Input: part model. Units: mm. Frame: model coordinates. Coordinates: 2 decimals unless noted, no trailing zeros. Order: outer loops, then holes, each group sorted by start corner. A loop starts at its lowest first (then second) coordinate and runs counter-clockwise, first axis right, second up. Notation, with made-up numbers: (52.25, 19.5) - (70.25, 19.5) arc R23 cw to (70.25, 27.5) - close; hole circle Ø2 at (15.5, 44.5). An arc over 180 degrees is marked (long way). One line per question, with ' | ' between items. Start each with the question number.
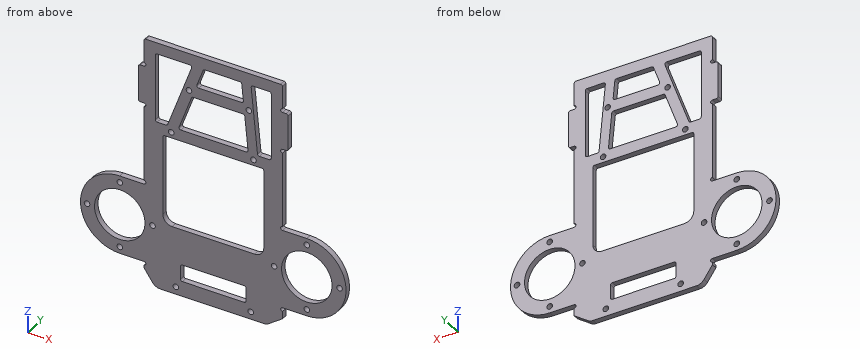
```python
from build123d import *
from OCP.BRepFilletAPI import BRepFilletAPI_MakeChamfer

# Parameters (mm, degrees)
SKETCH_1_R          = 13.5
SKETCH_1_R_2        = 1.5
EXTRUDE_1_DEPTH     = 3
SKETCH_3_W          = 54
SKETCH_3_H          = 48
SKETCH_3_W_2        = 35
SKETCH_3_H_2        = 9
CUT_EXTRUDE_2_DEPTH = 123.678441464
SKETCH_2_R          = 1
CUT_EXTRUDE_1_DEPTH = 123.678441464
CHAMFER_1_SIZE      = 6
CHAMFER_1_SIZE2     = 8.56888804
FILLET_1_R          = 1
FILLET_2_R          = 5


with BuildPart() as part:
    # 草图1 → 凸台-拉伸1 (new body)
    with BuildSketch(Plane(origin=(0, 0, 0), x_dir=(1, 0, 0), z_dir=(0, 1, 0))):
        with BuildLine():
            Line((-37, 21), (-50, 21))
            ThreePointArc((-50, 21), (-71, 0), (-50, -21))
            Line((-50, -21), (-37, -21))
            Line((-37, -21), (-37, -65))
            Line((-37, -65), (-40, -65))
            Line((-40, -65), (-40, -85))
            Line((-40, -85), (-37, -85))
            Line((-37, -85), (-37, -100))
            Line((-37, -100), (37, -100))
            Line((37, -100), (37, -85))
            Line((37, -85), (40, -85))
            Line((40, -85), (40, -65))
            Line((40, -65), (37, -65))
            Line((37, -65), (37, -21))
            Line((37, -21), (50, -21))
            ThreePointArc((50, -21), (71, 0), (50, 21))
            Line((50, 21), (37, 21))
            Line((37, 21), (37, 33))
            Line((37, 33), (-37, 33))
            Line((-37, 33), (-37, 21))
        make_face()
        with Locations(Location((-50, 0, 0), (0, 0, 270))):
            Circle(SKETCH_1_R, mode=Mode.SUBTRACT)
        with Locations(Location((50, 0, 0), (0, 0, 90))):
            Circle(SKETCH_1_R, mode=Mode.SUBTRACT)
        with Locations(Location((-50, 17.5, 0), (0, 0, 270))):
            Circle(SKETCH_1_R_2, mode=Mode.SUBTRACT)
        with Locations(Location((-32.5, 0, 0), (0, 0, 270))):
            Circle(SKETCH_1_R_2, mode=Mode.SUBTRACT)
        with Locations(Location((-67.5, 0, 0), (0, 0, 270))):
            Circle(SKETCH_1_R_2, mode=Mode.SUBTRACT)
        with Locations(Location((-50, -17.5, 0), (0, 0, 270))):
            Circle(SKETCH_1_R_2, mode=Mode.SUBTRACT)
        with Locations(Location((32.5, 0, 0), (0, 0, 270))):
            Circle(SKETCH_1_R_2, mode=Mode.SUBTRACT)
        with Locations(Location((50, -17.5, 0), (0, 0, 270))):
            Circle(SKETCH_1_R_2, mode=Mode.SUBTRACT)
        with Locations(Location((50, 17.5, 0), (0, 0, 270))):
            Circle(SKETCH_1_R_2, mode=Mode.SUBTRACT)
        with Locations(Location((67.5, 0, 0), (0, 0, 270))):
            Circle(SKETCH_1_R_2, mode=Mode.SUBTRACT)
        with Locations(Location((-20, 29, 0), (0, 0, 270))):
            Circle(SKETCH_1_R_2, mode=Mode.SUBTRACT)
        with Locations(Location((20, 29, 0), (0, 0, 90))):
            Circle(SKETCH_1_R_2, mode=Mode.SUBTRACT)
        with Locations(Location((21.5, -54, 0), (0, 0, 270))):
            Circle(SKETCH_1_R_2, mode=Mode.SUBTRACT)
        with Locations(Location((-13, -80, 0), (0, 0, 270))):
            Circle(SKETCH_1_R_2, mode=Mode.SUBTRACT)
        with Locations(Location((19, -80, 0), (0, 0, 270))):
            Circle(SKETCH_1_R_2, mode=Mode.SUBTRACT)
        with Locations(Location((-22.5, -54, 0), (0, 0, 270))):
            Circle(SKETCH_1_R_2, mode=Mode.SUBTRACT)
    extrude(amount=EXTRUDE_1_DEPTH)

    # 草图3 → 切除-拉伸2 (cut, through all)
    with BuildSketch(Plane(origin=(0, 3, 0), x_dir=(1, 0, 0), z_dir=(0, 1, 0))):
        with Locations((0, -27)):
            Rectangle(SKETCH_3_W, SKETCH_3_H)
        with Locations((0, 20.5)):
            Rectangle(SKETCH_3_W_2, SKETCH_3_H_2)
        Polygon((-24.597833201, -57), (-11.078602431, -94), (-31, -94), (-31, -57), align=None)
        Polygon((-18.742190282, -57), (18.700008099, -57), (16.776931176, -77), (-11.434497974, -77), align=None)
        Polygon((-9.242190282, -83), (-5.222959512, -94), (15.142315791, -94), (16.200008099, -83), align=None)
        Polygon((23.723068824, -57), (20.165376517, -94), (31, -94), (31, -57), align=None)
    extrude(amount=-CUT_EXTRUDE_2_DEPTH, mode=Mode.SUBTRACT)

    # 草图2 → 切除-拉伸1 (cut, through all)
    with BuildSketch(Plane(origin=(0, 3, 0), x_dir=(1, 0, 0), z_dir=(0, 1, 0))):
        with Locations((-37, 22)):
            Circle(SKETCH_2_R)
        with Locations((-37, -22)):
            Circle(SKETCH_2_R)
        with Locations((-37, -64)):
            Circle(SKETCH_2_R)
        with Locations((-37, -86)):
            Circle(SKETCH_2_R)
        with Locations((37, -86)):
            Circle(SKETCH_2_R)
        with Locations((37, -64)):
            Circle(SKETCH_2_R)
        with Locations((37, -22)):
            Circle(SKETCH_2_R)
        with Locations((37, 22)):
            Circle(SKETCH_2_R)
    extrude(amount=-CUT_EXTRUDE_1_DEPTH, mode=Mode.SUBTRACT)

    # 倒角1: one chamfer whose edges measure the first distance from different faces: ONE call of the kernel's chamfer builder (chamfer() names one face for all edges)
    chamfer_1_edges_1 = [part.edges().sort_by_distance(p)[0] for p in [
        (-37, 1.5, -33),
    ]]
    chamfer_1_side_1 = [part.faces().sort_by_distance(p)[0] for p in [
        (0, 1.5, -33),
    ]]
    chamfer_1_edges_2 = [part.edges().sort_by_distance(p)[0] for p in [
        (37, 1.5, -33),
    ]]
    chamfer_1_side_2 = [part.faces().sort_by_distance(p)[0] for p in [
        (37, 1.5, -28),
    ]]
    chamfer_1 = BRepFilletAPI_MakeChamfer(part.part.solid().wrapped)
    for e in chamfer_1_edges_1:
        chamfer_1.Add(CHAMFER_1_SIZE, CHAMFER_1_SIZE2, e.wrapped, chamfer_1_side_1[0].wrapped)  # the first distance lies on this face
    for e in chamfer_1_edges_2:
        chamfer_1.Add(CHAMFER_1_SIZE, CHAMFER_1_SIZE2, e.wrapped, chamfer_1_side_2[0].wrapped)  # the first distance lies on this face
    add(Compound.cast(chamfer_1.Shape()), mode=Mode.REPLACE)

    # 圆角1
    fillet_1_edges = [part.edges().sort_by_distance(p)[0] for p in [
        (23.723068824, 1.5, 57),
        (31, 1.5, 57),
        (31, 1.5, 94),
        (20.165376517, 1.5, 94),
        (-17.5, 1.5, -16),
        (-17.5, 1.5, -25),
        (17.5, 1.5, -25),
        (17.5, 1.5, -16),
        (-11.434497974, 1.5, 77),
        (-18.742190282, 1.5, 57),
        (18.700008099, 1.5, 57),
        (16.776931176, 1.5, 77),
        (-11.078602431, 1.5, 94),
        (-31, 1.5, 94),
        (-31, 1.5, 57),
        (-24.597833201, 1.5, 57),
        (-9.242190282, 1.5, 83),
        (16.200008099, 1.5, 83),
        (15.142315791, 1.5, 94),
        (-5.222959512, 1.5, 94),
        (-27, 1.5, 51),
        (27, 1.5, 51),
        (40, 1.5, 65),
        (40, 1.5, 85),
        (37, 1.5, 100),
        (-37, 1.5, 100),
        (-40, 1.5, 85),
        (-40, 1.5, 65),
    ]]
    fillet(fillet_1_edges, radius=FILLET_1_R)

    # 圆角2
    fillet_2_edges = [part.edges().sort_by_distance(p)[0] for p in [
        (-27, 1.5, 3),
        (27, 1.5, 3),
        (-31, 1.5, -33),
        (28.43111196, 1.5, -33),
    ]]
    fillet(fillet_2_edges, radius=FILLET_2_R)


solid = part.part
```
(1) Section A-A (z = 40). Output: boundary loops of the cut face in (x, y), then the cut area to 3 significant figures.
(2) Section B-B (x = -61). Output: boundary loops of the cut face in (y, z), then the cut area to 3 significant figures.
(3) Section D-D (y = 2.1). State how many separate pieces and enclosed holes the cut face has, then the cut area to 3 significant figures.
(4) Pin query (flat end, axial travel): pin 1 (1.5 mm diameter, centred on y = 1.5, z = 91, fed in from +X); pin 2 (0.9 mm diameter, centred on y = 1, z = 67.5, fed in from -X); pin 3 (0.6 mm diameter, centred on x = 38, y = 2, fed in from +Z). Return the tip coordinate at first contact, or that it passes through.
(5) Material intervals for line 1 along X through (y, z) = (0.5, 35); line 2 along X through (y, z) = (1.7, -17.5); line 3 along X through (y, z) = (0.8, 17.5), sorted ascending. Write a range as from..to.
(6) Section C-C (z = 5). Output: boundary loops of the cut face in (x, y).
Worked answers:
1) outline: (-37, 0) - (-27, 0) - (-27, 3) - (-37, 3) - close; (27, 0) - (37, 0) - (37, 3) - (27, 3) - close | area: 60.0 mm²
2) outline: (0, -17.89) - (3, -17.89) - (3, -7.83) - (0, -7.83) - close; (0, 7.83) - (3, 7.83) - (3, 17.89) - (0, 17.89) - close | area: 60.4 mm²
3) separate pieces: 1 | enclosed holes: 22 | area: 6,510 mm²
4) pin 1: stops at x = 37 | pin 2: stops at x = -40 | pin 3: stops at z = 85
5) line 1: x = -37..-27, 27..37 | line 2: x = -61.61..-51.5, -48.5..-17.5, 17.5..48.5, 51.5..61.61 | line 3: x = -61.61..-51.5, -48.5..-27, 27..48.5, 51.5..61.61
6) outline: (-70.4, 0) - (-62.54, 0) - (-62.54, 3) - (-70.4, 3) - close; (-37.46, 0) - (-26, 0) - (-26, 3) - (-37.46, 3) - close; (26, 0) - (37.46, 0) - (37.46, 3) - (26, 3) - close; (62.54, 0) - (70.4, 0) - (70.4, 3) - (62.54, 3) - close
